Can you work these out from the model? Positions are in its coordinate system, mm. A direction names the side the tool comes from. Give positions to 0.01 mm unless a question says otherwise; leave off trailing zeros. Write each loop counter-clockwise with the first axis right and the second up, starting at its lowest first coordinate (ties: lowest second). Pieces come first, ordered by that corner, then holes. Notation, with made-up numbers: (55, 22) -> (74, 22) arc R20 ccw to (74, 50) -> close; hole circle Ø11 at (76.25, 23). An arc over 180 degrees is marked (long way). One line per item, written item: value.
Autodesk Fusion 360 part; units mm, degrees
sketch "Sketch1" plane through (0, 0, 0) normal (0, 0, 1) x (1, 0, 0) in component "[a]_z_drive_baseplate_a_x2"
  line L0 (16.95, -21.4) -> (-16.95, -21.4)
  line L1 (-16.95, -21.4) -> (-16.95, 21.4)
  line L2 (-16.95, 21.4) -> (16.95, 21.4)
  line L3 (16.95, 21.4) -> (16.95, -21.4)
  line L4 (16.95, -21.4) -> (-16.95, 21.4) construction
  line L5 (-16.95, -21.4) -> (16.95, 21.4) construction
  circle A0 centre (0, 0) radius 2.7
  circle A1 centre (-12.15, 16.6) radius 3
  circle A2 centre (-12.15, 16.6) radius 1.7
  line L6 (4.2, 2.4249) -> (0, 4.8497)
  line L7 (0, 4.8497) -> (-4.2, 2.4249)
  line L8 (-4.2, 2.4249) -> (-4.2, -2.4249)
  line L9 (-4.2, -2.4249) -> (0, -4.8497)
  line L10 (0, -4.8497) -> (4.2, -2.4249)
  line L11 (4.2, -2.4249) -> (4.2, 2.4249)
  line L12 (0, -25) -> (0, 28) construction
  line L13 (-30, 0) -> (30, 0) construction
  circle A3 centre (12.15, 16.6) radius 3
  circle A4 centre (12.15, 16.6) radius 1.7
  circle A5 centre (12.15, -16.6) radius 3
  circle A6 centre (12.15, -16.6) radius 1.7
  circle A7 centre (0, 0) radius 4.1
  dimension "d1" = 33.9
  dimension "d2" = 42.8
  dimension "d3" = 5.4
  dimension "d4" = 6
  dimension "d5" = 4.8
  dimension "d6" = 4.8
  dimension "d7" = 3.4
  dimension "d8" = 4.2
  dimension "d18" = 8.2
extrude "Extrude1" add sketch "Sketch1" along normal mid plane 7 contours L0 L1 L2 L3 | A0 | A1 | A2 | L6 L7 L8 L9 L10 L11 | A3 | A4 | A5 | A6 | A7 in component "[a]_z_drive_baseplate_a_x2"
fillet "Fillet1" radius 3 4 edges at (16.95, -21.4, 0) (-16.95, -21.4, 0) (-16.95, 21.4, 0) (16.95, 21.4, 0) in component "[a]_z_drive_baseplate_a_x2"
extrude "Extrude2" cut sketch "Sketch1" along normal through all and the other way through all contours A0 | A2 | A4 | A6 in component "[a]_z_drive_baseplate_a_x2"
extrude "Extrude3" cut sketch "Sketch1" along normal through all from surface at 0.5 contours A1 | A2 | A3 | A4 | A5 | A6 in component "[a]_z_drive_baseplate_a_x2"
extrude "Extrude4" cut sketch "Sketch1" against normal through all from surface at 0.5 contours A0 | L6 L7 L8 L9 L10 L11 | A7 in component "[a]_z_drive_baseplate_a_x2"
sketch "Sketch2" plane through (0, 0, 0) normal (0, 0, 1) x (1, 0, 0) in component "[a]_z_drive_baseplate_a_x2"
sketch "Sketch3" plane through (0, 0, 0.5) normal (0, 0, -1) x (1, 0, 0) in component "[a]_z_drive_baseplate_a_x2"
  line L0 (4.2, -2.4249) -> (4.2, 2.4249)
  line L1 (4.2, 2.4249) -> (0, 4.8497)
  line L2 (0, 4.8497) -> (-4.2, 2.4249)
  line L3 (-4.2, 2.4249) -> (-4.2, -2.4249)
  line L4 (-4.2, -2.4249) -> (0, -4.8497)
  line L5 (0, -4.8497) -> (4.2, -2.4249)
  circle A0 centre (0, 0) radius 4.1
extrude "Extrude5" cut sketch "Sketch3" against normal through all draft -45 contours A0 in component "[a]_z_drive_baseplate_a_x2"
chamfer "Chamfer1" distance 0.4 angle 45 11 edges at (0, 21.4, -3.5) (16.0713, 20.5213, -3.5) (16.95, 0, -3.5) (16.0713, -20.5213, -3.5) (0, -21.4, -3.5) (-16.0713, -20.5213, -3.5) (-16.95, 0, -3.5) (-16.0713, 20.5213, -3.5) (10.565, 15.9853, -3.5) (10.565, -17.2147, -3.5) (-13.735, 15.9853, -3.5) in component "[a]_z_drive_baseplate_a_x2"
fillet "Fillet2" radius 1 8 edges at (16.0713, 20.5213, 3.5) (0, 21.4, 3.5) (-16.0713, 20.5213, 3.5) (-16.95, 0, 3.5) (-16.0713, -20.5213, 3.5) (0, -21.4, 3.5) (16.0713, -20.5213, 3.5) (16.95, 0, 3.5) in component "[a]_z_drive_baseplate_a_x2"
component "[a]_z_drive_baseplate_a_x2" placed x (1, 0, 0) y (0, 1, 0) z (0, 0, 1) at (0, 0, 0)
1) Will these pins go through, and if not, where does the flat tip stop? pin 1 (3 mm diameter, centred on x = -13, y = 16.5, fed in from +Z); pin 2 (3.5 mm diameter, centred on x = -12.15, y = 16.6, fed in from -Z); pin 3 (4 mm diameter, centred on x = -0.5, y = 1.5, fed in from -Z).
Answer list:
pin 1: stops at z = 0.5
pin 2: stops at z = -3.15
pin 3: stops at z = 1.02
2) We'd pull the mould along Y, two halves only. Please class faces 1 (the face through (10.45, -16.53, -1.27)), 2 (the face through (16.649, 0.258, 3.215)), 3 (the face through (0, 21.4, 0)): released by +Y, released by -Y, zero draft, split by the parting line, or undercut.
Answer list:
face 1: undercut
face 2: zero draft
face 3: released by +Y
3) I need wall thicknesses on L1, parallel to Y at x = 12.15, z = 1.95; L2, parallel to X at y = 16.6, z = 1.3; L3, parallel to X at y = 16.6, z = 2.65. Which ranges of each line are inside material? Lowest first, please.
Answer list:
L1: y = -21.4 to -19.6, -13.6 to 13.6, 19.6 to 21.4
L2: x = -16.95 to -15.15, -9.15 to 9.15, 15.15 to 16.95
L3: x = -16.94 to -15.15, -9.15 to 9.15, 15.15 to 16.94
4) If we section it at C-C (z = -1.5): Write out the boundary of the cut face in (x, y).
Answer list:
outline: (-16.95, -18.4) arc R3 ccw to (-13.95, -21.4) -> (13.95, -21.4) arc R3 ccw to (16.95, -18.4) -> (16.95, 18.4) arc R3 ccw to (13.95, 21.4) -> (-13.95, 21.4) arc R3 ccw to (-16.95, 18.4) -> close; hole circle Ø3.4 at (-12.15, 16.6); hole (-4.2, -2.42) -> (0, -4.85) -> (4.2, -2.42) -> (4.2, 2.42) -> (0, 4.85) -> (-4.2, 2.42) -> close; hole circle Ø3.4 at (12.15, -16.6); hole circle Ø3.4 at (12.15, 16.6)
5) If we section it at A-A (x = 12.15): Write out the boundary of the cut face in (y, z), and give its area (3 significant figures).
Answer list:
outline: (-21.4, -3.1) -> (-21, -3.5) -> (-18.7, -3.5) -> (-18.3, -3.1) -> (-18.3, 0.5) -> (-19.6, 0.5) -> (-19.6, 3.5) -> (-20.4, 3.5) arc R1 ccw to (-21.4, 2.5) -> close; (-14.9, -3.1) -> (-14.5, -3.5) -> (14.5, -3.5) -> (14.9, -3.1) -> (14.9, 0.5) -> (13.6, 0.5) -> (13.6, 3.5) -> (-13.6, 3.5) -> (-13.6, 0.5) -> (-14.9, 0.5) -> close; (18.3, -3.1) -> (18.7, -3.5) -> (21, -3.5) -> (21.4, -3.1) -> (21.4, 2.5) arc R1 ccw to (20.4, 3.5) -> (19.6, 3.5) -> (19.6, 0.5) -> (18.3, 0.5) -> close
area: 235 mm^2
6) If we section it at B-B (y = 0): Write out the boundary of the cut face in (x, z), and give its area (3 significant figures).
Answer list:
outline: (-16.95, -3.1) -> (-16.55, -3.5) -> (-4.2, -3.5) -> (-4.2, 0.5) -> (-4.1, 0.5) -> (-2.7, 1.9) -> (-2.7, 3.5) -> (-15.95, 3.5) arc R1 ccw to (-16.95, 2.5) -> close; (2.7, 1.9) -> (4.1, 0.5) -> (4.2, 0.5) -> (4.2, -3.5) -> (16.55, -3.5) -> (16.95, -3.1) -> (16.95, 2.5) arc R1 ccw to (15.95, 3.5) -> (2.7, 3.5) -> close
area: 185 mm^2
7) If we section it at D-D (x = -12.15): Write out the boundary of the cut face in (y, z).
Answer list:
outline: (-21.4, -3.1) -> (-21, -3.5) -> (14.5, -3.5) -> (14.9, -3.1) -> (14.9, 0.5) -> (13.6, 0.5) -> (13.6, 3.5) -> (-20.4, 3.5) arc R1 ccw to (-21.4, 2.5) -> close; (18.3, -3.1) -> (18.7, -3.5) -> (21, -3.5) -> (21.4, -3.1) -> (21.4, 2.5) arc R1 ccw to (20.4, 3.5) -> (19.6, 3.5) -> (19.6, 0.5) -> (18.3, 0.5) -> close
8) For faces 4 (the face through (-2.13, -3.62, -1.47)), 5 (the face through (15.89, 20.298, -3.386)), 6 (the face through (14, 17, 0.5)), which set-ups out of +Z, -Z, +X, -X, +Y, -Y let a thin tool reach every point of the face, with its end or its side?
Answer list:
face 4: -Z
face 5: -Z, +X, +Y
face 6: +Z
